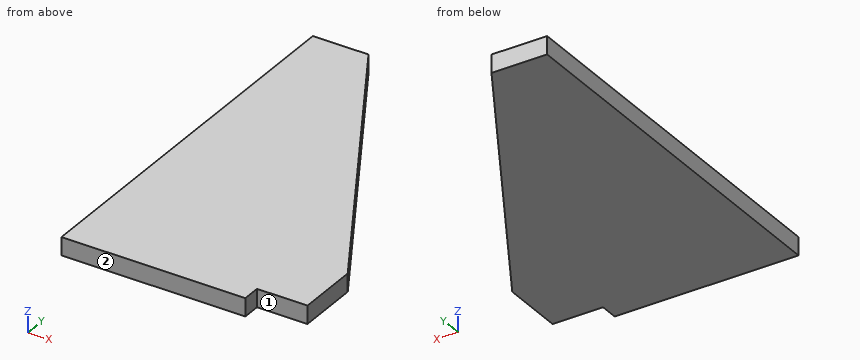
Autodesk Inventor part; units mm, degrees
ref_plane "YZ Plane" through (0, 0, 0) normal (1, 0, 0) x (0, 1, 0)
ref_plane "XZ Plane" through (0, 0, 0) normal (0, 1, 0) x (-1, 0, 0)
ref_plane "XY Plane" through (0, 0, 0) normal (0, 0, 1) x (1, 0, 0)
sketch "Sketch3" plane through (0, 0, 0) normal (0, 0, 1) x (1, 0, 0)
  line L0 (0, 0) -> (-150, 0)
  line L1 (-150, 0) -> (-150, 10)
  line L2 (-150, 10) -> (0, 10)
  line L3 (0, 10) -> (0, 0)
  line L4 (0, 10) -> (-150, 269.8076)
  line L5 (-150, 269.8076) -> (-150, 10)
  line L6 (-20, 44.641) -> (-20, 10)
  line L7 (-48, 0) -> (-48, 93.1384)
  line L8 (-150, 216.3134) -> (-119.1151, 216.3134)
  point P0 (-48, 10)
  dimension "d19" = 150
  dimension "d29" = 10
  dimension "d31" = 60
  dimension "d32" = 20
  dimension "d34" = 48
extrude "Plate3" add sketch "Sketch3" along normal blind 10 contours L0 L1 L2 L7 | L7 L4 L6 L2 | L2 L5 L8 L4 L7
equation "\"d18\" = Thickness"
equation "\"BendReliefDepth\" = 0.5 * Thickness"
properties part number "NVPH-319 conductor"
Work out the finished part from the listing and answer in its coordinate system (mm). Face numbers are marked on the shaded views. A direction names the side the tool comes from. Round coordinates to 2 decimals unless told otherwise and drop trailing zeros. Loops run counter-clockwise (first coordinate to the right, second up) from the corner with the lowest first, then second, coordinate; pieces in that order, holes last. Notation, with made-up numbers: (46, 89.25) -> (94, 89.25) arc R15 cw to (94, 107.25) -> close; hole circle Ø7 at (82, 83). An arc over 180 degrees is marked (long way). Use one line per item in the form item = value.
(1) Find section C-C on x = -87. Give the vertices of the cut face in (y, z), then the cut area to 3 significant figures.
Answer list:
outline = (0, 0) -> (160.69, 0) -> (160.69, 10) -> (0, 10) -> close
area = 1,610 mm2
(2) Straight lines are drawn through the part: line 1 (Y direction, x = -26.5, z = 4); line 2 (X direction, y = 124, z = 1.25); line 3 (X direction, y = 119.5, z = 6.5). For each, find the intervals that lie inside material, in ascending order.
Answer list:
line_1 = 10 to 55.9
line_2 = -150 to -65.82
line_3 = -150 to -63.22
(3) Flat-ended cylindrical pins translate along their axes: P1, Ø5, axis at x = -97, z = 1.5, coming from the +Y side; P2, Ø6, axis at y = 149.5, z = 6.5, coming from the +X side. Find the tip coordinate at first contact, or state that the pin passes through.
Answer list:
P1 = 182.34
P2 = -78.81
(4) Find section B-B on y = 191. Give the vertices of the cut face in (x, z).
Answer list:
outline = (-150, 0) -> (-104.5, 0) -> (-104.5, 10) -> (-150, 10) -> close
(5) A tool of negligible diameter and unlimited length cuts with its end or side. For the marked faces 1 and 2, from which of +Z, -Z, +X, -X, +Y, -Y can it reach the whole face along a straight path? Write none if from no direction.
Answer list:
face_1 = +Z, -Z, +X, -Y
face_2 = +Z, -Z, +X, -X, -Y
(6) Find section A-A on z = 5. Give the vertices of the cut face in (x, y), then the cut area to 3 significant figures.
Answer list:
outline = (-150, 0) -> (-48, 0) -> (-48, 10) -> (-20, 10) -> (-20, 44.64) -> (-119.12, 216.31) -> (-150, 216.31) -> close
area = 19,300 mm2
